Geometry check sheet. Reference: the model listing, model coordinates, mm. Give positions to 0.01 mm unless a question says otherwise; leave off trailing zeros. Loops run counter-clockwise (first coordinate to the right, second up) from the corner with the lowest first, then second, coordinate; pieces in that order, holes last. Notation, with made-up numbers: (48.5, 48) -> (67.5, 48) arc R20 ccw to (67.5, 58) -> close; hole circle Ø5 at (82, -24). An arc over 180 degrees is marked (long way). One line per item, written item: value. Start each with the question number.
(1) Scan lines: line 1 along X through (y, z) = (100, 644); line 2 along Y through (x, z) = (-11.5, 365.5); line 3 along X through (y, z) = (110, 275). Record each from-to range of solid material in increasing order. Write a range as from..to.
(2) Sectioned sample at A-A, the plane z = 265.5. Record the cut outline in (x, y), then the cut area to 3 significant figures.
(3) Sectioned sample at B-B, the plane x = 42.5. Record the cut outline in (y, z).
(4) Gauge pin test, flat ends, axial feed: pin 1 Ø3 at (y, z) = (109.5, 325) entering from +X; pin 2 Ø12 at (x, z) = (44, 213.5) entering from -Y; pin 3 Ø12 at (x, z) = (3, 464.5) entering from -Y. Record the tip position at first contact, or that the pin passes through.
Autodesk Inventor part; units mm, degrees
ref_plane "YZ Plane" through (0, 0, 0) normal (1, 0, 0) x (0, 1, 0)
ref_plane "XZ Plane" through (0, 0, 0) normal (0, 1, 0) x (-1, 0, 0)
ref_plane "XY Plane" through (0, 0, 0) normal (0, 0, 1) x (1, 0, 0)
sketch "Sketch1" plane through (0, 0, 0) normal (0, 0, 1) x (1, 0, 0)
  line L0 (0, 0) -> (0, 132.08)
  line L1 (0, 132.08) -> (25.4, 132.08)
  line L2 (0, 66.04) -> (63.5, 66.04)
  line L3 (0, 132.08) -> (0, 66.04)
  line L4 (0, 99.06) -> (31.75, 99.06)
  arc A0 (63.5, 99.06) -> (55.043838, 120.634513) centre (31.75, 99.06) ccw
  line L5 (0, 66.04) -> (0, 0)
  arc A1 (54.194148, 10.562869) -> (63.5, 33.02) centre (31.75, 33.02) ccw
  line L6 (63.5, 28.211314) -> (63.5, 99.06)
  arc A2 (59.079555, 115.220381) -> (25.4, 132.08) centre (28.846947, 96.896052) ccw
  line L7 (0, 0) -> (25.4, 0)
  arc A3 (25.4, 0) -> (63.5, 28.211314) centre (28.813006, 35.223762) ccw
  line L8 (0, 132.08) -> (-25.4, 132.08)
  line L9 (0, 1.27) -> (0, 132.08)
  line L10 (0, 132.08) -> (-25.4, 132.08)
  line L11 (-25.4, 132.08) -> (-25.4, 1.27)
  line L12 (-25.4, 0) -> (0, 0)
  line L13 (0, 0) -> (0, 132.08)
  line L14 (0, 132.08) -> (-25.4, 132.08)
  line L15 (-25.4, 132.08) -> (-25.4, 0)
  dimension "d0" = 132.08
  dimension "d1" = 25.4
  dimension "d2" = 63.5
  dimension "d3" = 25.4
  dimension "d4" = 25.4
sketch "Sketch1 outline for Extrusion1" plane through (0, 0, 0) normal (0, 0, 1) x (1, 0, 0)
  line L0 (-25.4, 0) -> (25.4, 0)
  arc A0 (25.4, 0) -> (63.5, 28.211314) centre (28.813006, 35.223762) ccw
  line L1 (63.5, 28.211314) -> (63.5, 99.06)
  arc A1 (63.5, 99.06) -> (59.079555, 115.220381) centre (31.75, 99.06) ccw
  arc A2 (59.079555, 115.220381) -> (25.4, 132.08) centre (28.846947, 96.896052) ccw
  line L2 (25.4, 132.08) -> (-25.4, 132.08)
  line L3 (-25.4, 132.08) -> (-25.4, 0)
extrude "Extrusion1" add sketch "Sketch1 outline for Extrusion1" along normal blind 774.7
properties part number "Chassis_Bumper(29in)"
Calculated:
1. line 1: x = -25.4..63.49
1. line 2: y = 0..132.08
1. line 3: x = -25.4..61.56
2. outline: (-25.4, 0) -> (25.4, 0) arc R35.39 ccw to (63.5, 28.21) -> (63.5, 99.06) arc R31.75 ccw to (59.08, 115.22) arc R35.35 ccw to (25.4, 132.08) -> (-25.4, 132.08) -> close
2. area: 11,300 mm2
3. outline: (2.59, 0) -> (129.51, 0) -> (129.51, 774.7) -> (2.59, 774.7) -> close
4. pin 1: stops at x = 62.22
4. pin 2: stops at y = 1.05
4. pin 3: stops at y = 0
